Print and shaded views of the part. All mm, measured from the part's lowest x, y and z. A direction names the side the tool comes from. Give positions to 0.01 mm unless a question says otherwise; leave off trailing zeros. Order: outer loops, then holes, each group sorted by start corner. A loop starts at its lowest first (then second) coordinate and runs counter-clockwise, first axis right, second up. Notation, with made-up numbers: (34, 48) -> (40, 48) arc R31 cw to (40, 76) -> close; hole circle Ø5 at (-31, 60.25). An arc over 180 degrees is marked (long way). One line per question, with ' | ' between items. Start each with the question number.
(1) Cut at C-C (z = 8.75). Give the cut face in (x, y).
(2) Cut at A-A (x = 33). Give the cut face in (y, z) (1 decimal).
(3) Drill centre lines: L1, parallel to X at y = 24.25, z = 9; L2, parallel to X at y = 4.25, z = 13; L3, parallel to Z at x = 46.5, y = 21.5. Where is each one in solid material? Low to high. Write a range as from..to.
(4) Pull direction Z, two halves, no side cores. Call the marked faces 5, 6 and 7: +Z half, -Z half, draft (parallel to the pull), parting line (faces both ways), or undercut.
(5) Pin check, flat tips, straight feed: pin 1 Ø4 at (y, z) = (6, 5.5) entering from -X; pin 2 Ø2.5 at (x, y) = (45, 21) entering from +Z; pin 3 Ø7.5 at (x, y) = (5, 9) entering from +Z; pin 4 Ø2 at (x, y) = (15, 18.5) entering from +Z (1 decimal). Stop position of each tip, or through.
(6) Which spindle directions (+Z, -Z, +X, -X, +Y, -Y) get a long thin tool onto all of the face, cutting with end or side? Do the marked faces 1, 2, 3 and 4. Say none if no direction does.
(7) Cut at B-B (y = 22.25). Give the cut face in (x, z) (1 decimal), then the cut area to 3 significant figures.
(8) Cut at D-D (y = 1.5). Give the cut face in (x, z).
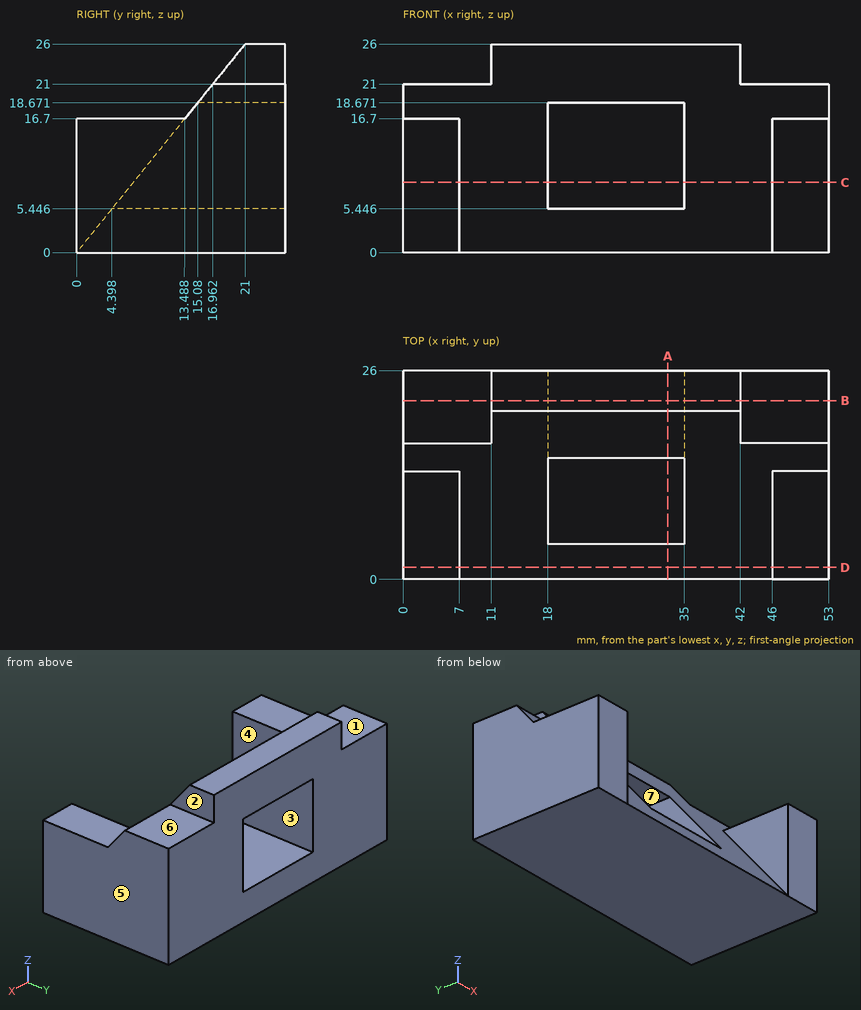
Result set:
1) outline: (0, 0) -> (7, 0) -> (7, 7.07) -> (18, 7.07) -> (18, 26) -> (0, 26) -> close; (35, 7.07) -> (46, 7.07) -> (46, 0) -> (53, 0) -> (53, 26) -> (35, 26) -> close
2) outline: (0, 0) -> (26, 0) -> (26, 5.4) -> (4.4, 5.4) -> close; (15.1, 18.7) -> (26, 18.7) -> (26, 26) -> (21, 26) -> close
3) L1: x = 0..18, 35..53 | L2: x = 0..7, 46..53 | L3: z = 0..21
4) face 5: draft | face 6: +Z half | face 7: undercut
5) pin 1: stops at x = 0 | pin 2: stops at z = 21 | pin 3: stops at z = 16.7 | pin 4: stops at z = 24.1
6) face 1: +Z, -X, +Y, -Y | face 2: +Z, +X, +Y, -Y | face 3: +Y, -Y | face 4: +Z, -Y
7) outline: (0, 0) -> (53, 0) -> (53, 21) -> (42, 21) -> (42, 26) -> (11, 26) -> (11, 21) -> (0, 21) -> close; hole (18, 5.4) -> (35, 5.4) -> (35, 18.7) -> (18, 18.7) -> close | area: 1,040 mm2
8) outline: (0, 0) -> (53, 0) -> (53, 16.7) -> (46, 16.7) -> (46, 1.86) -> (7, 1.86) -> (7, 16.7) -> (0, 16.7) -> close
